Verification items for the finished model (mm, model axes). Face numbers are marked on the shaded views. Give positions to 0.01 mm unless a question says otherwise; leave off trailing zeros. Write each loop counter-clockwise with the first axis right and the second up, starting at its lowest first coordinate (ties: lowest second). Pieces come first, ordered by that corner, then holes. Notation, with made-up numbers: M 81,49.25 L 99,49.25 A38 ccw 99,87.25 Z; hole C 50,54.5 d7. An arc over 180 degrees is marked long. Answer as a JSON object with one key per item and string values.
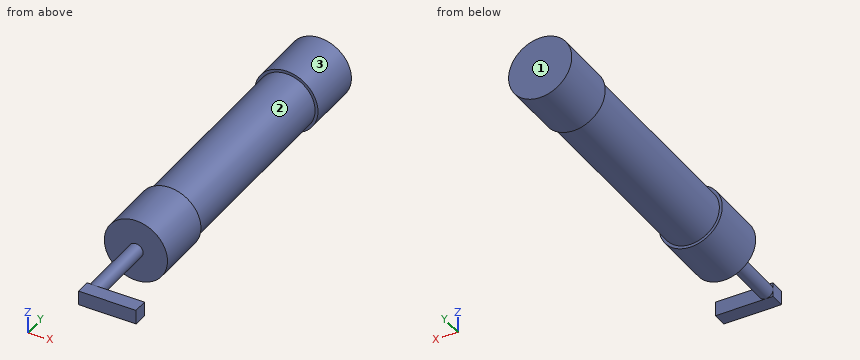
Autodesk Inventor part; units mm, degrees
ref_plane "YZ Plane" through (0, 0, 0) normal (1, 0, 0) x (0, 1, 0)
ref_plane "XZ Plane" through (0, 0, 0) normal (0, 1, 0) x (-1, 0, 0)
ref_plane "XY Plane" through (0, 0, 0) normal (0, 0, 1) x (1, 0, 0)
sketch "Эскиз1" plane through (0, 0, 0) normal (0, 1, 0) x (-1, 0, 0)
  circle A0 centre (0, 0) radius 10
  dimension "d0" = 20
extrude "Выдавливание1" add sketch "Эскиз1" along normal blind 70
thread "Резьба2"
sketch "Эскиз2" plane through (0, 70, 0) normal (0, 1, 0) x (1, 0, 0)
  point P0 (0, 0)
sketch "Эскиз3" plane through (0, 70, 0) normal (0, 1, 0) x (1, 0, 0)
  circle A0 centre (0, 0) radius 11
  dimension "d7" = 22
extrude "Выдавливание2" add sketch "Эскиз3" along normal blind 20
sketch "Эскиз6" plane through (0, 0, 0) normal (0, -1, 0) x (1, 0, 0)
  circle A0 centre (0, 0) radius 11
extrude "Выдавливание5" add sketch "Эскиз6" along normal blind 20
sketch "Эскиз7" plane through (0, -20, 0) normal (0, -1, 0) x (1, 0, 0)
  circle A0 centre (0, 0) radius 2.5
  dimension "d18" = 5
extrude "Выдавливание6" add sketch "Эскиз7" along normal blind 30
sketch "Эскиз8" plane through (0, -50, 0) normal (0, -1, 0) x (1, 0, 0)
  line L0 (-2.5, 2.5) -> (-2.5, 0)
  line L1 (17.5, -2.5) -> (17.5, 2.5)
  line L2 (-2.5, 2.5) -> (17.5, 2.5)
  line L3 (17.5, 2.5) -> (17.5, -2.5)
  line L4 (17.5, -2.5) -> (-2.5, -2.5)
  line L5 (-2.5, -2.5) -> (-2.5, 2.5)
  point P0 (0, 0)
extrude "Выдавливание7" add sketch "Эскиз8" against normal blind 5
properties part number "Вал штурвала"
1) Thickness scan on L1, parallel to Y at x = 2, z = -4.25; L2, parallel to Y at x = 7.75, z = -1.5; L3, parallel to X at y = 29, z = -6.75. Record the ranges inside material, lowest first.
Completed:
{"L1": "y = -20 to 90", "L2": "y = -50 to -45, -20 to 90", "L3": "x = -7.38 to 7.38"}
2) Release check for a two-part mould opening along Y. For the marked faces 1, 2 and 3 record: pulls with the +Y half, pulls with the -Y half, needs draft (parallel to the pull), parting line crosses it, or undercut.
Completed:
{"face 1": "pulls with the +Y half", "face 2": "undercut", "face 3": "needs draft"}
3) Section check B-B on x = -4.5. Record the boundary of the cut face in (y, z).
Completed:
{"outline": "M -20,-10.04 L 0,-10.04 L 0,-8.93 L 70,-8.93 L 70,-10.04 L 90,-10.04 L 90,10.04 L 70,10.04 L 70,8.93 L 0,8.93 L 0,10.04 L -20,10.04 Z"}
4) Section check D-D on z = 1.25. Record the boundary of the cut face in (x, y), and give its area (3 significant figures).
Completed:
{"outline": "M -10.93,-20 L -2.17,-20 L -2.17,-45 L -2.5,-45 L -2.5,-50 L 17.5,-50 L 17.5,-45 L 2.17,-45 L 2.17,-20 L 10.93,-20 L 10.93,0 L 9.92,0 L 9.92,70 L 10.93,70 L 10.93,90 L -10.93,90 L -10.93,70 L -9.92,70 L -9.92,0 L -10.93,0 Z", "area": "2,470 mm2"}
5) Go/stop test with flat-tipped pins: pin 1 (1 mm diameter, centred on y = 7.5, z = -6, fed in from -X); pin 2 (1.5 mm diameter, centred on y = -47.5, z = -0.5, fed in from -X); pin 3 (6 mm diameter, centred on y = 23, z = 3.5, fed in from -X); pin 4 (4 mm diameter, centred on x = 13.5, z = -6.5, fed in from +Y). Record where each tip stops, or that it passes through.
Completed:
{"pin 1": "stops at x = -8.35", "pin 2": "stops at x = -2.5", "pin 3": "stops at x = -9.99", "pin 4": "passes through"}
6) Section check A-A on z = 8.75. Record the boundary of the cut face in (x, y).
Completed:
{"outline": "M -6.67,-20 L 6.67,-20 L 6.67,0 L 4.84,0 L 4.84,70 L 6.67,70 L 6.67,90 L -6.67,90 L -6.67,70 L -4.84,70 L -4.84,0 L -6.67,0 Z"}
7) Section check C-C on y = 59. Record the boundary of the cut face in (x, z).
Completed:
{"outline": "C 0,0 d20"}
